Can you work these out from the model? Positions are in its coordinate system, mm. Face numbers are marked on the shaded views. A direction names the side the tool comes from. Give positions to 0.01 mm unless a question says otherwise; leave off trailing zeros. Loops run counter-clockwise (first coordinate to the right, second up) from the corner with the lowest first, then second, coordinate; pieces in that order, holes last. Notation, with made-up numbers: M 37.5,52.25 L 63.5,52.25 A22 cw 63.5,90.25 Z; hole C 25,30 d2. An arc over 180 degrees is marked long. One line per item, written item: value. Start each with the question number.
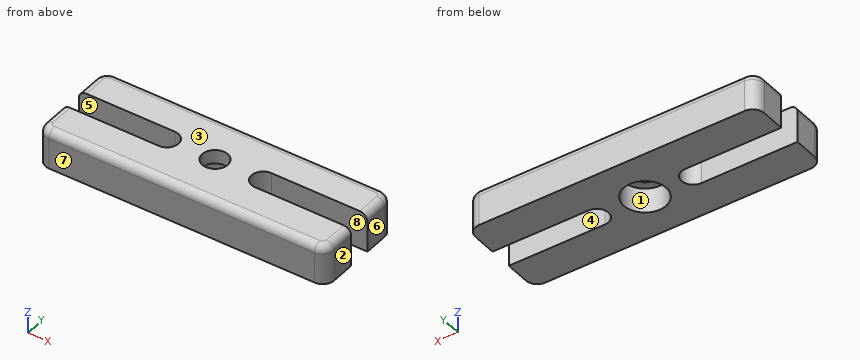
from build123d import *

# Parameters (mm, degrees)
PAD_DEPTH        = 10
HOLE_D           = 6.6
HOLE_DEPTH       = 25
HOLE_CBORE_D     = 11
HOLE_CBORE_DEPTH = 6.4
FILLET_R         = 2
FILLET001_R      = 2


with BuildPart() as part:
    # Sketch → Pad (new body)
    with BuildSketch(Plane.XY):
        with BuildLine():
            Line((-34.5, 12.25), (34.5, 12.25))
            ThreePointArc((37.5, 9.25), (36.62132, 11.37132), (34.5, 12.25))
            Line((37.5, 9.25), (37.5, 3))
            Line((37.5, 3), (12.5, 3))
            ThreePointArc((12.5, 3), (9.5, 0), (12.5, -3))
            Line((12.5, -3), (37.5, -3))
            Line((37.5, -3), (37.5, -9.25))
            ThreePointArc((34.5, -12.25), (36.62132, -11.37132), (37.5, -9.25))
            Line((34.5, -12.25), (-34.5, -12.25))
            ThreePointArc((-37.5, -9.25), (-36.62132, -11.37132), (-34.5, -12.25))
            Line((-37.5, -9.25), (-37.5, -3))
            Line((-37.5, -3), (-12.5, -3))
            ThreePointArc((-12.5, -3), (-9.5, 0), (-12.5, 3))
            Line((-12.5, 3), (-37.5, 3))
            Line((-37.5, 3), (-37.5, 9.25))
            ThreePointArc((-34.5, 12.25), (-36.62132, 11.37132), (-37.5, 9.25))
        make_face()
    extrude(amount=PAD_DEPTH)

    # Hole
    with Locations(Plane(origin=(0, 0, 0), x_dir=(1, 0, 0), z_dir=(0, 0, -1))):
        with Locations((0, 0)):
            CounterBoreHole(HOLE_D / 2, HOLE_CBORE_D / 2, HOLE_CBORE_DEPTH, depth=HOLE_DEPTH)

    # Fillet
    fillet_edges = [part.edges().sort_by_distance(p)[0] for p in [
        (0, 12.25, 10),
    ]]
    fillet(fillet_edges, radius=FILLET_R)

    # Fillet001
    fillet001_edges = [part.edges().sort_by_distance(p)[0] for p in [
        (0, -12.25, 10),
    ]]
    fillet(fillet001_edges, radius=FILLET001_R)


solid = part.part
Q1. If we section it at B-B, the plane z = 4: Write out the boundary of the cut face in (x, y).
Q2. If we section it at A-A, the plane y = 0: Write out the boundary of the cut face in (x, z), plus the area to 3 significant figures.
Q3. If we section it at D-D, the plane x = 23: Write out the boundary of the cut face in (y, z).
Q4. If we mould it in two halves opening along Y, with no side actions, what happens to the marked faces 6, 7 and 8? For each: released by +Y, released by -Y, zero draft, split by the parting line, or undercut.
Q5. I need wall thicknesses on line 1 along Y through (x, z) = (0, 4.5); line 2 along Y through (x, z) = (-30, 4); line 3 along X through (y, z) = (2.5, 2.75). Which ranges of each line are inside material? Lowest first, please.
Q6. If we section it at C-C, the plane x = 0: Write out the boundary of the cut face in (y, z).
Q7. For P1, Ø12.5, axis at x = 0, y = 0, coming from the -Z side, with a flat end and sliding along its axis, tell me the tip position at first contact or that it passes through.
Q8. Which directions (+Z, -Z, +X, -X, +Y, -Y) give clear straight access to the entire face, cutting with the end or side of a thin tool? Please do the marked faces 1, 2, 3, 4 and 5.
Response:
1. outline: M -37.5,-9.25 A3 ccw -34.5,-12.25 L 34.5,-12.25 A3 ccw 37.5,-9.25 L 37.5,-3 L 12.5,-3 A3 cw 12.5,3 L 37.5,3 L 37.5,9.25 A3 ccw 34.5,12.25 L -34.5,12.25 A3 ccw -37.5,9.25 L -37.5,3 L -12.5,3 A3 cw -12.5,-3 L -37.5,-3 Z; hole C 0,0 d11
2. outline: M -9.5,0 L -5.5,0 L -5.5,6.4 L -3.3,6.4 L -3.3,10 L -9.5,10 Z; M 3.3,6.4 L 5.5,6.4 L 5.5,0 L 9.5,0 L 9.5,10 L 3.3,10 Z
2. area: 95.8 mm^2
3. outline: M -12.25,0 L -3,0 L -3,10 L -10.25,10 A2 ccw -12.25,8 Z; M 3,0 L 12.25,0 L 12.25,8 A2 ccw 10.25,10 L 3,10 Z
4. face 6: zero draft
4. face 7: released by -Y
4. face 8: undercut
5. line 1: -12.25 to -5.5, 5.5 to 12.25
5. line 2: -12.25 to -3, 3 to 12.25
5. line 3: -10.84 to -4.9, 4.9 to 10.84
6. outline: M -12.25,0 L -5.5,0 L -5.5,6.4 L -3.3,6.4 L -3.3,10 L -10.25,10 A2 ccw -12.25,8 Z; M 3.3,6.4 L 5.5,6.4 L 5.5,0 L 12.25,0 L 12.25,8 A2 ccw 10.25,10 L 3.3,10 Z
7. P1: z = 0
8. face 1: -Z
8. face 2: +Z, -Z, +X, +Y, -Y
8. face 3: +Z, +X, -X, +Y, -Y
8. face 4: +Z, -Z, +X
8. face 5: +Z, -Z, -X
